Geometry check sheet. Reference: the model listing, model coordinates, mm. Coordinates: 2 decimals unless noted, no trailing zeros. Order: outer loops, then holes, each group sorted by start corner. A loop starts at its lowest first (then second) coordinate and runs counter-clockwise, first axis right, second up. Notation, with made-up numbers: (20.25, 41.25) - (67.25, 41.25) arc R27 ccw to (67.25, 58.25) - close; hole circle Ø3 at (6.25, 72). An arc over 180 degrees is marked (long way). One line per item, written item: value. Start each with the question number.
```python
from build123d import *

# Parameters (mm, degrees)
SKETCH1_W           = 200
SKETCH1_H           = 160
SKETCH1_W_2         = 292.37604307
SKETCH1_H_2         = 30
BOSS_EXTRUDE1_DEPTH = 2
SKETCH2_R           = 4
SKETCH2_R_2         = 11
SKETCH2_R_3         = 1.5
CUT_EXTRUDE1_DEPTH  = 3
SKETCH4_W           = 292.37604307
SKETCH4_H           = 50
BOSS_EXTRUDE2_DEPTH = 2
FILLET1_R           = 10
SKETCH5_R           = 1.5
SKETCH5_W           = 60
SKETCH5_H           = 32
CUT_EXTRUDE2_DEPTH  = 11


with BuildPart() as part:
    # Sketch1 → Boss-Extrude1 (new body)
    with BuildSketch(Plane.XY):
        Rectangle(SKETCH1_W, SKETCH1_H)
        Polygon((192.37604307, 80), (100, -80), (100, 80), align=None)
        with Locations((46.188021535, 95)):
            Rectangle(SKETCH1_W_2, SKETCH1_H_2)
    extrude(amount=BOSS_EXTRUDE1_DEPTH)

    # Sketch2 → Cut-Extrude1 (cut)
    with BuildSketch(Plane.XY.offset(2)):
        with Locations((93.07179677, -68)):
            Circle(SKETCH2_R)
        with Locations((177.364936071, 78)):
            Circle(SKETCH2_R)
        with Locations((-67, 22)):
            Circle(SKETCH2_R_2)
        with Locations((-75, -68)):
            Circle(SKETCH2_R)
        with Locations((-53, 22)):
            Circle(SKETCH2_R_3)
        with Locations((-67, 36)):
            Circle(SKETCH2_R_3)
        with Locations((-81, 22)):
            Circle(SKETCH2_R_3)
        with Locations((-67, 8)):
            Circle(SKETCH2_R_3)
        with Locations((54.54952947, -67.242640687)):
            Circle(SKETCH2_R_3)
        with Locations((63.034810844, -58.757359313)):
            Circle(SKETCH2_R_3)
        with Locations((14.225855729, -60.5)):
            Circle(SKETCH2_R_3)
        with Locations((-40.127135228, -67.242640687)):
            Circle(SKETCH2_R_3)
        with Locations((-31.641853854, -58.757359313)):
            Circle(SKETCH2_R_3)
        with Locations((-90.295627115, 102.881439108)):
            Circle(SKETCH2_R_3)
        with Locations((-73.186266887, 96.138798421)):
            Circle(SKETCH2_R_3)
        with Locations((-64.700985513, 104.624079796)):
            Circle(SKETCH2_R_3)
        with Locations((15.078196993, 96.138798421)):
            Circle(SKETCH2_R_3)
        with Locations((23.563478368, 104.624079796)):
            Circle(SKETCH2_R_3)
        with Locations((41.969500075, 33.138798421)):
            Circle(SKETCH2_R_3)
        with Locations((50.454781449, 41.624079796)):
            Circle(SKETCH2_R_3)
        with Locations((116.811272287, 33.138798421)):
            Circle(SKETCH2_R_3)
        with Locations((125.296553661, 41.624079796)):
            Circle(SKETCH2_R_3)
        with Locations((14.225855729, 25)):
            Circle(SKETCH2_R)
        with Locations((176.305585362, 125.488938255)):
            Circle(SKETCH2_R_3)
        with Locations((-55.814717647, 143.138798421)):
            Circle(SKETCH2_R_3)
        with Locations((-47.329436273, 151.624079796)):
            Circle(SKETCH2_R_3)
        with Locations((111.655390934, 143.138798421)):
            Circle(SKETCH2_R_3)
        with Locations((120.140672308, 151.624079796)):
            Circle(SKETCH2_R_3)
        with Locations((-17.947932492, -69.117445741)):
            Circle(SKETCH2_R)
        with Locations((37.494421294, -69.117445741)):
            Circle(SKETCH2_R)
        with BuildLine():
            Line((75.290389443, 11.241781095), (75.290389443, 37.908558601))
            ThreePointArc((75.290389443, 37.908558601), (79.290389443, 41.908558601), (83.290389443, 37.908558601))
            Line((83.290389443, 37.908558601), (83.290389443, 11.241781095))
            ThreePointArc((83.290389443, 11.241781095), (79.290389443, 7.241781095), (75.290389443, 11.241781095))
        make_face()
        with BuildLine():
            Line((-72, 82), (-47, 82))
            ThreePointArc((-47, 82), (-43, 78), (-47, 74))
            Line((-47, 74), (-72, 74))
            ThreePointArc((-72, 74), (-76, 78), (-72, 82))
        make_face()
    extrude(amount=-CUT_EXTRUDE1_DEPTH, mode=Mode.SUBTRACT)

    # Sketch4 → Boss-Extrude2 (add)
    with BuildSketch(Plane.XY.offset(2)):
        with Locations((46.188021535, 135)):
            Rectangle(SKETCH4_W, SKETCH4_H)
    extrude(amount=-BOSS_EXTRUDE2_DEPTH)

    # Fillet1
    fillet1_edges = [part.edges().sort_by_distance(p)[0] for p in [
        (-100, 160, 1),
        (192.37604307, 160, 1),
        (-100, -80, 1),
        (192.37604307, 80, 1),
        (100, -80, 1),
    ]]
    fillet(fillet1_edges, radius=FILLET1_R)

    # Sketch5 → Cut-Extrude2 (cut)
    with BuildSketch(Plane.XY.offset(2)):
        with Locations((-55.814717647, 143.138798421)):
            Circle(SKETCH5_R)
        with Locations((-47.329436273, 151.624079796)):
            Circle(SKETCH5_R)
        with Locations((111.655390934, 143.138798421)):
            Circle(SKETCH5_R)
        with Locations((120.140672308, 151.624079796)):
            Circle(SKETCH5_R)
        with Locations((176.305585362, 125.488938255)):
            Circle(SKETCH5_R)
        with Locations((-16.178132997, 129.381439108)):
            Rectangle(SKETCH5_W, SKETCH5_H)
    extrude(amount=-CUT_EXTRUDE2_DEPTH, mode=Mode.SUBTRACT)


solid = part.part
```
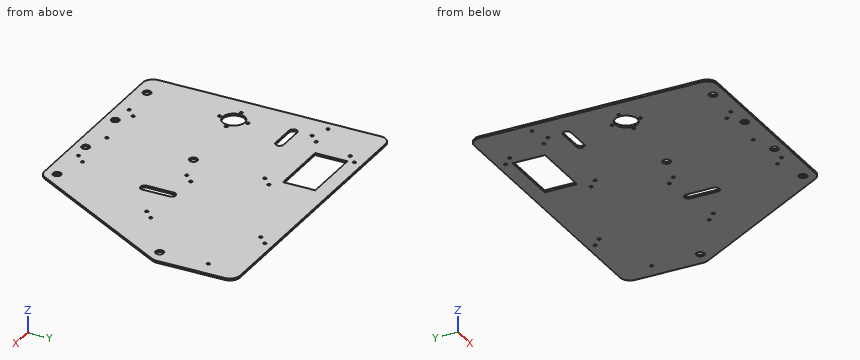
Q1. Cross-section at D-D, the plane y = -10. Enter the section's corners in (x, z).
Q2. Cross-section at C-C, the plane x = 163. Enter the section's corners in (y, z).
Q3. Gauge pin test, flat ends, axial feed: P1, Ø4, axis at x = -47.33, y = 151.62, coming from the -Z side; P2, Ø0.6, axis at y = 23, z = 1.5, coming from the +X side. Record the tip position at first contact, or that the pin passes through.
Q4. Cross-section at B-B, the plane z = 0.7. Count the separate pieces of the cut face and the enclosed holes in it, and give its area (3 significant figures).
Q5. Material ranges on probe 1 along Y at (x, z) = (-67, 1.5); probe 2 along X at (y, z) = (8.5, 1.4); probe 3 along X at (y, z) = (128, 0.3), recorded low to high.
Q6. Cross-section at A-A, the plane y = 133. Enter the section's corners in (x, z).
Check result:
1. outline: (-100, 0) - (140.41, 0) - (140.41, 2) - (-100, 2) - close
2. outline: (29.12, 0) - (160, 0) - (160, 2) - (29.12, 2) - close
3. P1: stops at z = 0
3. P2: stops at x = 159.64
4. separate pieces: 1
4. enclosed holes: 33
4. area: 59,400 mm2
5. probe 1: y = -80 to 6.5, 9.5 to 11, 33 to 34.5, 37.5 to 74, 82 to 160
5. probe 2: x = -100 to -68.41, -65.59 to 76.38, 82.2 to 151.1
5. probe 3: x = -100 to -46.18, 13.82 to 192.38
6. outline: (-100, 0) - (-46.18, 0) - (-46.18, 2) - (-100, 2) - close; (13.82, 0) - (192.38, 0) - (192.38, 2) - (13.82, 2) - close
